from build123d import *

# Parameters (mm, degrees)
SOCKET_CUT_EXTRUDE1_START  = -3.54
SOCKET_CUT_EXTRUDE1_DEPTH  = 3.54
SKETCH13_R                 = 3
LENGTH_BOSS_EXTRUDE1_DEPTH = 20


with BuildPart() as part:
    # Sketch8 → Head-Revolve1 (revolve)
    with BuildSketch(Plane(origin=(0, 0, 0), x_dir=(0, 0, -1), z_dir=(1, 0, 0))):
        with BuildLine():
            Line((-4.4, 4.75), (-4.4, 2.8))
            Line((-4.4, 2.8), (-4.189927833, 2.016))
            Line((-4.189927833, 2.016), (-4.189927833, 0))
            Line((-4.189927833, 0), (0, 0))
            Line((0, 0), (0, 5))
            Line((0, 5), (-4.15, 5))
            ThreePointArc((-4.15, 5), (-4.326776695, 4.926776695), (-4.4, 4.75))
        make_face()
    revolve(axis=Axis((0, 0, 0), (0, 0, 1)))

    # Sketch9 → socket-Cut-Extrude1 (cut)
    with BuildSketch(Plane.XY.offset(4.4).offset(SOCKET_CUT_EXTRUDE1_START)):
        with BuildLine():
            ThreePointArc((0.544244974, 2.369331508), (1.008, 1.745907214), (1.779778789, 1.655995727))
            ThreePointArc((1.779778789, 1.655995727), (2.424871131, 1.4), (2.324023763, 0.713335781))
            ThreePointArc((2.324023763, 0.713335781), (2.016, 0), (2.324023763, -0.713335781))
            ThreePointArc((2.324023763, -0.713335781), (2.424871131, -1.4), (1.779778789, -1.655995727))
            ThreePointArc((1.779778789, -1.655995727), (1.008, -1.745907214), (0.544244974, -2.369331508))
            ThreePointArc((0.544244974, -2.369331508), (0, -2.8), (-0.544244974, -2.369331508))
            ThreePointArc((-0.544244974, -2.369331508), (-1.008, -1.745907214), (-1.779778789, -1.655995727))
            ThreePointArc((-1.779778789, -1.655995727), (-2.424871131, -1.4), (-2.324023763, -0.713335781))
            ThreePointArc((-2.324023763, -0.713335781), (-2.016, 0), (-2.324023763, 0.713335781))
            ThreePointArc((-2.324023763, 0.713335781), (-2.424871131, 1.4), (-1.779778789, 1.655995727))
            ThreePointArc((-1.779778789, 1.655995727), (-1.008, 1.745907214), (-0.544244974, 2.369331508))
            ThreePointArc((-0.544244974, 2.369331508), (0, 2.8), (0.544244974, 2.369331508))
        make_face()
    extrude(amount=SOCKET_CUT_EXTRUDE1_DEPTH, mode=Mode.SUBTRACT)

    # Sketch12 → Socket-Revolve2 (revolve)
    with BuildSketch(Plane(origin=(0, 0, 0), x_dir=(0, 0, -1), z_dir=(1, 0, 0)), mode=Mode.PRIVATE) as socket_revolve2_sk:
        Polygon((-2.11, 5), (-2.11, 2.8), (-0.86, 0), (0, 0), (0, 5), align=None)
    revolve(socket_revolve2_sk.sketch.rotate(Axis((0, 0, 0), (0, 0, -1)), 90), axis=Axis((0, 0, 0), (0, 0, -1)))

    # Sketch13 → Length-Boss-Extrude1 (add)
    with BuildSketch(Plane.XY):
        Circle(SKETCH13_R)
    extrude(amount=-LENGTH_BOSS_EXTRUDE1_DEPTH)

    # Sketch14 → Runout-Cut-Revolve1 (revolve, cut)
    with BuildSketch(Plane(origin=(0, 0, 0), x_dir=(0, 0, -1), z_dir=(1, 0, 0)), mode=Mode.PRIVATE) as runout_cut_revolve1_sk:
        Polygon((0, 3), (2, 3), (1, 2.675), (0, 2.675), align=None)
    revolve(runout_cut_revolve1_sk.sketch.rotate(Axis((0, 0, 0), (0, 0, -1)), 90), axis=Axis((0, 0, 0), (0, 0, -1)), mode=Mode.SUBTRACT)

    # Sketch15 → Fillet-Revolve3 (revolve)
    with BuildSketch(Plane(origin=(0, 0, 0), x_dir=(0, 0, -1), z_dir=(1, 0, 0)), mode=Mode.PRIVATE) as fillet_revolve3_sk:
        with BuildLine():
            ThreePointArc((0.146390721, 3.0375), (0.536304234, 2.769379359), (1, 2.675))
            Line((1, 2.675), (0, 2.675))
            Line((0, 2.675), (0, 3.4))
            ThreePointArc((0, 3.4), (0.037979272, 3.204528459), (0.146390721, 3.0375))
        make_face()
    revolve(fillet_revolve3_sk.sketch.rotate(Axis((0, 0, 0), (0, 0, -1)), 90), axis=Axis((0, 0, 0), (0, 0, -1)))

    # Sketch16 → Chamfer-Cut-Revolve2 (revolve, cut)
    with BuildSketch(Plane(origin=(0, 0, 0), x_dir=(0, 0, -1), z_dir=(1, 0, 0)), mode=Mode.PRIVATE) as chamfer_cut_revolve2_sk:
        Polygon((20, 3), (19.268859171, 3), (20, 2.3865), align=None)
    revolve(chamfer_cut_revolve2_sk.sketch.rotate(Axis((0, 0, 0), (0, 0, -1)), 90), axis=Axis((0, 0, 0), (0, 0, -1)), mode=Mode.SUBTRACT)


solid = part.part
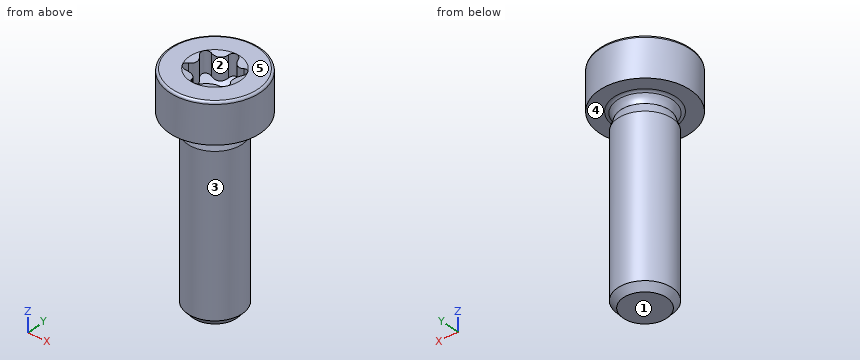
Could you check a few things on this model? Use its own coordinates, in mm. Face numbers are marked on the shaded views. A direction names the side the tool comes from. Coordinates: 2 decimals unless noted, no trailing zeros. Write each loop counter-clockwise with the first axis right and the second up, starting at its lowest first coordinate (ties: lowest second). Pieces come first, ordered by that corner, then holes. Notation, with made-up numbers: M 14,62.25 L 39,62.25 A26 cw 39,94.25 Z; hole C 76,-13 d3. An arc over 180 degrees is marked long. One line per question, with ' | ' between items.
1) For pin 1 Ø6 at (y, z) = (-3.5, -2) entering from -X; pin 2 Ø3 at (x, y) = (-1, 0.5) entering from +Z; pin 3 Ø1.5 at (x, z) = (3.5, 0) entering from +Y, each with a flat end and sliding along its axis, tell me the tip position at first contact or that it passes through.
Checks:
pin 1: x = -4.84 | pin 2: z = 4.35 | pin 3: y = 4.18
2) I need wall thicknesses on probe 1 along Z at (x, y) = (-3.75, -2); probe 2 along X at (y, z) = (-0.25, 0.5); probe 3 along Y at (x, z) = (0, -19). Which ranges of each line are inside material? Lowest first, please. Write a range as [from, to].
Checks:
probe 1: [0, 4.4] | probe 2: [-4.99, 4.99] | probe 3: [-3, 3]
3) Imagine slicing it at A-A, the plane z = -7.75. Write out the boundary of the cut face in (x, y), and give its area (3 significant figures).
Checks:
outline: C 0,0 d6 | area: 28.3 mm²
4) If we mould it in two halves opening along X, with no side actions, what happens to the marked faces 1, 2 and 3? For each: released by +X, released by -X, zero draft, split by the parting line, or undercut.
Checks:
face 1: zero draft | face 2: undercut | face 3: split by the parting line
5) For the marked faces 4 and 5, which set-ups out of +Z, -Z, +X, -X, +Y, -Y let a thin tool reach every point of the face, with its end or its side?
Checks:
face 4: -Z | face 5: +Z, +X, -X, +Y, -Y
6) Imagine slicing it at B-B, the plane z = 0.5. Write out the boundary of the cut face in (x, y).
Checks:
outline: C 0,0 d10
